Autodesk Inventor part; units mm, degrees
ref_plane "p_XY" through (0, 0, 0) normal (0, 1, 0) x (1, 0, 0)
ref_plane "p_YZ" through (0, 0, 0) normal (1, 0, 0) x (0, 0, -1)
ref_plane "p_ZX" through (0, 0, 0) normal (0, 0, -1) x (0, 1, 0)
sketch "Sketch_1" plane through (0, 0, 0) normal (0, 0, 1) x (1, 0, 0)
  line L0 (-18.75, -12.5) -> (-17, -12.5)
  line L1 (-17, -12.5) -> (-17, -7.2)
  line L2 (-17, -7.2) -> (17, -7.2)
  line L3 (17, -7.2) -> (17, -12.5)
  line L4 (17, -12.5) -> (18.75, -12.5)
  line L5 (18.75, -12.5) -> (18.75, 0)
  line L6 (18.75, 0) -> (14, 0)
  line L7 (14, 0) -> (14, 12.5)
  line L8 (14, 12.5) -> (11, 12.5)
  line L9 (11, 12.5) -> (11, 0)
  line L10 (11, 0) -> (-18.75, 0)
  line L11 (-18.75, 0) -> (-18.75, -12.5)
extrude "Extrusion1" add sketch "Sketch_1" along normal blind 178
sketch "Sketch_2" plane through (-18.75, 0, 0) normal (0, 1, 0) x (0, 0, 1)
  line L0 (6.645, 11.65) -> (28.795, 11.65)
  line L1 (28.795, 11.65) -> (28.795, 25.85)
  line L2 (28.795, 25.85) -> (6.645, 25.85)
  line L3 (6.645, 25.85) -> (6.645, 11.65)
extrude "Extrusion2" cut sketch "Sketch_2" against normal blind 8
sketch "Sketch_3" plane through (-18.75, 0, 0) normal (0, 1, 0) x (0, 0, 1)
  line L0 (42.355, 25.85) -> (42.355, 11.65)
  line L1 (42.355, 11.65) -> (64.505, 11.65)
  line L2 (64.505, 11.65) -> (64.505, 25.85)
  line L3 (64.505, 25.85) -> (42.355, 25.85)
extrude "Extrusion3" cut sketch "Sketch_3" against normal blind 8
sketch "Sketch_4" plane through (-18.75, 0, 0) normal (0, 1, 0) x (0, 0, 1)
  line L0 (78.065, 11.65) -> (100.215, 11.65)
  line L1 (100.215, 11.65) -> (100.215, 25.85)
  line L2 (100.215, 25.85) -> (78.065, 25.85)
  line L3 (78.065, 25.85) -> (78.065, 11.65)
extrude "Extrusion4" cut sketch "Sketch_4" against normal blind 8
sketch "Sketch_5" plane through (-18.75, 0, 0) normal (0, 1, 0) x (0, 0, 1)
  line L0 (113.775, 25.85) -> (113.775, 11.65)
  line L1 (113.775, 11.65) -> (135.925, 11.65)
  line L2 (135.925, 11.65) -> (135.925, 25.85)
  line L3 (135.925, 25.85) -> (113.775, 25.85)
extrude "Extrusion5" cut sketch "Sketch_5" against normal blind 8
sketch "Sketch_6" plane through (-18.75, 0, 0) normal (0, 1, 0) x (0, 0, 1)
  line L0 (149.485, 25.85) -> (149.485, 11.65)
  line L1 (149.485, 11.65) -> (171.635, 11.65)
  line L2 (171.635, 11.65) -> (171.635, 25.85)
  line L3 (171.635, 25.85) -> (149.485, 25.85)
extrude "Extrusion6" cut sketch "Sketch_6" against normal blind 8
sketch "Sketch_10" plane through (-18.75, -12.5, 0) normal (-1, 0, 0) x (0, 0, 1)
  line L0 (27.9, 10) -> (27.9, 0)
  line L1 (27.9, 0) -> (43.3, 0)
  line L2 (43.3, 0) -> (43.3, 10)
  line L3 (43.3, 10) -> (27.9, 10)
extrude "Extrusion7" cut sketch "Sketch_10" against normal blind 37.5
sketch "Sketch_13" plane through (-17, -7.2, 0) normal (0, -1, 0) x (1, 0, 0)
  line L0 (0, 175) -> (0, 3)
  line L1 (0, 3) -> (34, 3)
  line L2 (34, 3) -> (34, 175)
  line L3 (34, 175) -> (0, 175)
extrude "Extrusion8" cut sketch "Sketch_13" against normal blind 4.7
ref_plane "p_XY" through (0, 0, 0) normal (0, 1, 0) x (1, 0, 0)
ref_plane "p_YZ" through (0, 0, 0) normal (1, 0, 0) x (0, 0, -1)
ref_plane "p_ZX" through (0, 0, 0) normal (0, 0, -1) x (0, 1, 0)
ref_plane "p1_XY" through (0, -9.5, 17.72) normal (1, 0, 0) x (0, 0, -1)
ref_plane "p1_YZ" through (0, -9.5, 17.72) normal (0, 0, -1) x (0, 1, 0)
ref_plane "p1_ZX" through (0, -9.5, 17.72) normal (0, 1, 0) x (1, 0, 0)
ref_plane "p2_XY" through (0, -9.5, 53.43) normal (1, 0, 0) x (0, 0, -1)
ref_plane "p2_YZ" through (0, -9.5, 53.43) normal (0, 0, -1) x (0, 1, 0)
ref_plane "p2_ZX" through (0, -9.5, 53.43) normal (0, 1, 0) x (1, 0, 0)
ref_plane "p3_XY" through (0, -9.5, 89.14) normal (1, 0, 0) x (0, 0, -1)
ref_plane "p3_YZ" through (0, -9.5, 89.14) normal (0, 0, -1) x (0, 1, 0)
ref_plane "p3_ZX" through (0, -9.5, 89.14) normal (0, 1, 0) x (1, 0, 0)
ref_plane "p4_XY" through (0, -9.5, 124.85) normal (1, 0, 0) x (0, 0, -1)
ref_plane "p4_YZ" through (0, -9.5, 124.85) normal (0, 0, -1) x (0, 1, 0)
ref_plane "p4_ZX" through (0, -9.5, 124.85) normal (0, 1, 0) x (1, 0, 0)
ref_plane "p5_XY" through (0, -9.5, 160.56) normal (1, 0, 0) x (0, 0, -1)
ref_plane "p5_YZ" through (0, -9.5, 160.56) normal (0, 0, -1) x (0, 1, 0)
ref_plane "p5_ZX" through (0, -9.5, 160.56) normal (0, 1, 0) x (1, 0, 0)
ref_plane "p6_XY" through (0, -9.5, 196.27) normal (1, 0, 0) x (0, 0, -1)
ref_plane "p6_YZ" through (0, -9.5, 196.27) normal (0, 0, -1) x (0, 1, 0)
ref_plane "p6_ZX" through (0, -9.5, 196.27) normal (0, 1, 0) x (1, 0, 0)
ref_plane "p7_XY" through (0, -9.5, 231.98) normal (1, 0, 0) x (0, 0, -1)
ref_plane "p7_YZ" through (0, -9.5, 231.98) normal (0, 0, -1) x (0, 1, 0)
ref_plane "p7_ZX" through (0, -9.5, 231.98) normal (0, 1, 0) x (1, 0, 0)
properties part number "PRO10282 Rollenleiste Abdeckung mit Seitenfuehrung 178"
Geometry check sheet. Reference: the model listing, model coordinates, mm. A direction names the side the tool comes from. Give positions to 0.01 mm unless a question says otherwise; leave off trailing zeros. Write each loop counter-clockwise with the first axis right and the second up, starting at its lowest first coordinate (ties: lowest second). Pieces come first, ordered by that corner, then holes. Notation, with made-up numbers: (24.5, 23.25) -> (43.5, 23.25) arc R24 cw to (43.5, 50.25) -> close; hole circle Ø1 at (59.5, 76.25). An arc over 180 degrees is marked (long way). Use one line per item in the form item = value.
Item 1: Mould release check, pull along Y, two halves, no side actions. Record for faces 1 (the flat face through (0, -7.2, 176)), 2 (the flat face through (11, 6, 88)), 3 (the flat face through (13, 12.5, 88)): released by +Y, released by -Y, zero draft, split by the parting line, or undercut.
Results list:
face_1 = released by -Y
face_2 = zero draft
face_3 = released by +Y
Item 2: Scan lines: line 1 (X direction, y = -8.75, z = 58); line 2 (Z direction, x = -7, y = -4.75); line 3 (Z direction, x = -3, y = -0.75) (3 decimals). Record each from-to range of solid material in increasing order.
Results list:
line_1 = -18.75 to -17, 17 to 18.75
line_2 = 0 to 3, 175 to 178
line_3 = 0 to 6.645, 28.795 to 42.355, 64.505 to 78.065, 100.215 to 113.775, 135.925 to 149.485, 171.635 to 178
Item 3: Depth check by flat-ended pin: pin 1 Ø11 at (x, z) = (-9.5, 127) entering from -Y; pin 2 Ø2 at (x, y) = (1.5, -8.5) entering from -Z; pin 3 Ø5 at (x, z) = (-6.5, 32) entering from +Y; pin 4 Ø4 at (y, z) = (8.5, 106) entering from +X. Enter the tip coordinate at first touch or a pass-through.
Results list:
pin_1 = -2.5
pin_2 = through
pin_3 = 0
pin_4 = 14
Item 4: Sectioned sample at B-B on y = -9. Enter the section's corners in (x, z), plus the area to 3 significant figures.
Results list:
outline = (-18.75, 0) -> (-17, 0) -> (-17, 27.9) -> (-18.75, 27.9) -> close; (-18.75, 43.3) -> (-17, 43.3) -> (-17, 178) -> (-18.75, 178) -> close; (17, 0) -> (18.75, 0) -> (18.75, 27.9) -> (17, 27.9) -> close; (17, 43.3) -> (18.75, 43.3) -> (18.75, 178) -> (17, 178) -> close
area = 569 mm2
Item 5: Sectioned sample at A-A on z = 165.5. Enter the section's corners in (x, y).
Results list:
outline = (-18.75, -12.5) -> (-17, -12.5) -> (-17, -2.5) -> (-7.1, -2.5) -> (-7.1, 0) -> (-18.75, 0) -> close; (7.1, -2.5) -> (17, -2.5) -> (17, -12.5) -> (18.75, -12.5) -> (18.75, 0) -> (14, 0) -> (14, 12.5) -> (11, 12.5) -> (11, 0) -> (7.1, 0) -> close
Item 6: Access from +Z, -Z, +X, -X, +Y, -Y to the whole of each face (thin tool, end or side, straight path). Record for faces 4 (the flat face through (16, 0, 88)), 5 (the flat face through (-10, 0, 88)), 6 (the flat face through (0, -7.2, 1)), 7 (the flat face through (-17, -8, 112)).
Results list:
face_4 = +Z, -Z, +X, +Y
face_5 = +Z, -Z, -X, +Y
face_6 = +Z, -Z, -Y
face_7 = -Y
Item 7: Sectioned sample at D-D on x = -11.5. Enter the section's corners in (y, z).
Results list:
outline = (-7.2, 0) -> (0, 0) -> (0, 178) -> (-7.2, 178) -> (-7.2, 175) -> (-2.5, 175) -> (-2.5, 3) -> (-7.2, 3) -> close
Item 8: Sectioned sample at C-C on x = -1.5. Enter the section's corners in (y, z) (3 decimals), plus the area to 3 significant figures.
Results list:
outline = (-7.2, 0) -> (0, 0) -> (0, 6.645) -> (-2.5, 6.645) -> (-2.5, 3) -> (-7.2, 3) -> close; (-7.2, 175) -> (-2.5, 175) -> (-2.5, 171.635) -> (0, 171.635) -> (0, 178) -> (-7.2, 178) -> close; (-2.5, 28.795) -> (0, 28.795) -> (0, 42.355) -> (-2.5, 42.355) -> close; (-2.5, 64.505) -> (0, 64.505) -> (0, 78.065) -> (-2.5, 78.065) -> close; (-2.5, 100.215) -> (0, 100.215) -> (0, 113.775) -> (-2.5, 113.775) -> close; (-2.5, 135.925) -> (0, 135.925) -> (0, 149.485) -> (-2.5, 149.485) -> close
area = 196 mm2
